Verification items for the finished model (mm, model axes). Face numbers are marked on the shaded views. A direction names the side the tool comes from. Coordinates: 2 decimals unless noted, no trailing zeros. Write each loop counter-clockwise with the first axis right and the second up, starting at its lowest first coordinate (ties: lowest second). Pieces come first, ordered by that corner, then holes. Notation, with made-up numbers: (-29, 44) -> (-2, 44) arc R15 cw to (-2, 73) -> close; hole circle Ø9 at (-36, -13). An arc over 180 degrees is marked (long way). Answer in a Markdown table with one row per item.
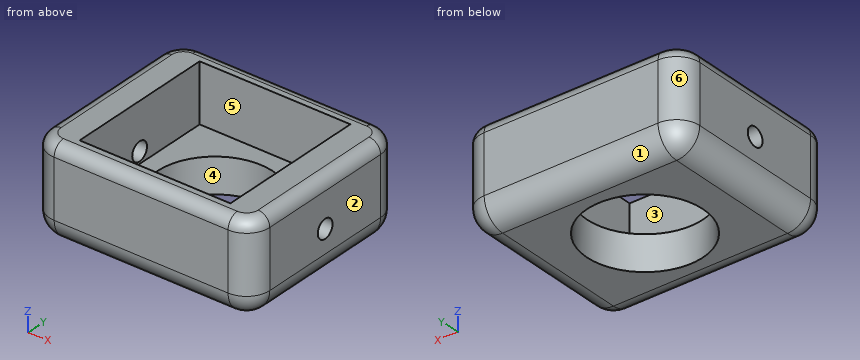
```python
from build123d import *

# Parameters (mm, degrees)
F0_W         = 19
F0_H         = 16
F0_W_2       = 13
F0_H_2       = 13
F0_R         = 5
F1_DEPTH     = 3
F2_W         = 19
F2_H         = 16
F2_W_2       = 13
F2_H_2       = 13
F3_DEPTH     = 5
F5_D         = 1.6
F6_R         = 2
F7_T1_DEPTH  = 11
F7_S5_W      = 2
F7_S5_H      = 2
F7_T6_DEPTH  = 2
F7_S11_W     = 2
F7_S11_H     = 2
F7_T12_DEPTH = 2
F7_S17_W     = 2
F7_S17_H     = 2
F7_T18_DEPTH = 2
F7_S23_W     = 2
F7_S23_H     = 2
F7_T24_DEPTH = 2
F8_R         = 1


# Not quite as in the source:
# - a fillet or chamfer that OpenCascade refuses, or shapes differently, is made with other operations: its cross-section is extruded or revolved along the edge and cut away or added


with BuildPart() as f1:
    # F0 (on Top) → F1 (new body)
    with BuildSketch(Plane.XY):
        Rectangle(F0_W, F0_H)
        Rectangle(F0_W_2, F0_H_2, mode=Mode.SUBTRACT)
        Rectangle(F0_W_2, F0_H_2)
        Circle(F0_R, mode=Mode.SUBTRACT)
    extrude(amount=F1_DEPTH)

    # F2 (on face) → F3 (join)
    with BuildSketch(Plane.XY.offset(3)):
        Rectangle(F2_W, F2_H)
        Rectangle(F2_W_2, F2_H_2, mode=Mode.SUBTRACT)
    extrude(amount=F3_DEPTH)

    # F5 (through all)
    with Locations(Plane.YZ.offset(9.5)):
        with Locations((0, 4)):
            Hole(F5_D / 2)

    # F6
    f6_edges = [f1.edges().sort_by_distance(p)[0] for p in [
        (0, -8, 0),
        (0, 8, 0),
        (-9.5, 0, 0),
        (9.5, 0, 0),
    ]]
    fillet(f6_edges, radius=F6_R)

    # F7: fillet of radius 2 on 4 edges, made by hand

    # F7_s2 → F7_t1 (cut)
    with BuildSketch(Plane.XY.offset(2)):
        with BuildLine():
            ThreePointArc((9.5, -6), (8.9142135624, -7.4142135624), (7.5, -8))
            Line((7.5, -8), (9.5, -8))
            Line((9.5, -8), (9.5, -6))
        make_face()
        with BuildLine():
            ThreePointArc((9.5, 6), (8.9142135624, 7.4142135624), (7.5, 8))
            Line((7.5, 8), (9.5, 8))
            Line((9.5, 8), (9.5, 6))
        make_face()
        with BuildLine():
            ThreePointArc((-7.5, -8), (-8.9142135624, -7.4142135624), (-9.5, -6))
            Line((-9.5, -6), (-9.5, -8))
            Line((-9.5, -8), (-7.5, -8))
        make_face()
        with BuildLine():
            ThreePointArc((-7.5, 8), (-8.9142135624, 7.4142135624), (-9.5, 6))
            Line((-9.5, 6), (-9.5, 8))
            Line((-9.5, 8), (-7.5, 8))
        make_face()
    extrude(amount=F7_T1_DEPTH, mode=Mode.SUBTRACT)


with BuildPart() as f7_tool4:
    # F7_s5 → F7_t6 (new body)
    with BuildSketch(Plane.XZ.offset(-6)):
        with Locations((-8.5, 1)):
            Rectangle(F7_S5_W, F7_S5_H)
    extrude(amount=-F7_T6_DEPTH)

    # F7_s7 → F7_t8 (revolve, cut)
    with BuildSketch(Plane(origin=(-7.5, 6, 2), x_dir=(0.7071067812, 0, 0.7071067812), z_dir=(-0.7071067812, 0, 0.7071067812))):
        with BuildLine():
            ThreePointArc((0, -2), (2, 0), (0, 2))
            Line((0, 2), (0, -2))
        make_face()
    revolve(axis=Axis((-7.5, 6, 2), (0, 1, 0)), mode=Mode.SUBTRACT)


with BuildPart() as f1_1:
    add(f1.part)

    # F7_t3: cut F7_tool4
    add(f7_tool4.part, mode=Mode.SUBTRACT)


with BuildPart() as f7_tool10:
    # F7_s11 → F7_t12 (new body)
    with BuildSketch(Plane.XZ.offset(6)):
        with Locations((-8.5, 1)):
            Rectangle(F7_S11_W, F7_S11_H)
    extrude(amount=F7_T12_DEPTH)

    # F7_s13 → F7_t14 (revolve, cut)
    with BuildSketch(Plane(origin=(-7.5, -6, 2), x_dir=(0.7071067812, 0, 0.7071067812), z_dir=(0.7071067812, 0, -0.7071067812))):
        with BuildLine():
            ThreePointArc((0, -2), (2, 0), (0, 2))
            Line((0, 2), (0, -2))
        make_face()
    revolve(axis=Axis((-7.5, -6, 2), (0, -1, 0)), mode=Mode.SUBTRACT)


with BuildPart() as f1_2:
    add(f1_1.part)

    # F7_t9: cut F7_tool10
    add(f7_tool10.part, mode=Mode.SUBTRACT)


with BuildPart() as f7_tool16:
    # F7_s17 → F7_t18 (new body)
    with BuildSketch(Plane.YZ.offset(7.5)):
        with Locations((7, 1)):
            Rectangle(F7_S17_W, F7_S17_H)
    extrude(amount=F7_T18_DEPTH)

    # F7_s19 → F7_t20 (revolve, cut)
    with BuildSketch(Plane(origin=(7.5, 6, 2), x_dir=(0, -0.7071067812, 0.7071067812), z_dir=(0, 0.7071067812, 0.7071067812))):
        with BuildLine():
            ThreePointArc((0, -2), (2, 0), (0, 2))
            Line((0, 2), (0, -2))
        make_face()
    revolve(axis=Axis((7.5, 6, 2), (1, 0, 0)), mode=Mode.SUBTRACT)


with BuildPart() as f1_3:
    add(f1_2.part)

    # F7_t15: cut F7_tool16
    add(f7_tool16.part, mode=Mode.SUBTRACT)


with BuildPart() as f7_tool22:
    # F7_s23 → F7_t24 (new body)
    with BuildSketch(Plane.YZ.offset(7.5)):
        with Locations((-7, 1)):
            Rectangle(F7_S23_W, F7_S23_H)
    extrude(amount=F7_T24_DEPTH)

    # F7_s25 → F7_t26 (revolve, cut)
    with BuildSketch(Plane(origin=(7.5, -6, 2), x_dir=(0, 0.7071067812, 0.7071067812), z_dir=(0, 0.7071067812, -0.7071067812))):
        with BuildLine():
            ThreePointArc((0, -2), (2, 0), (0, 2))
            Line((0, 2), (0, -2))
        make_face()
    revolve(axis=Axis((7.5, -6, 2), (1, 0, 0)), mode=Mode.SUBTRACT)


with BuildPart() as f1_4:
    add(f1_3.part)

    # F7_t21: cut F7_tool22
    add(f7_tool22.part, mode=Mode.SUBTRACT)

    # F8
    f8_edges = [f1_4.edges().sort_by_distance(p)[0] for p in [
        (0, 8, 8),
    ]]
    fillet(f8_edges, radius=F8_R)


solid = f1_4.part
```
1. Section check C-C, the plane x = 0. Record the boundary of the cut face in (y, z), plus the area to 3 significant figures.
Geometry says:
| item | result |
|---|---|
| outline | (-8, 2) arc R2 ccw to (-6, 0) -> (-5, 0) -> (-5, 3) -> (-6.5, 3) -> (-6.5, 8) -> (-7, 8) arc R1 ccw to (-8, 7) -> close; (5, 0) -> (6, 0) arc R2 ccw to (8, 2) -> (8, 7) arc R1 ccw to (7, 8) -> (6.5, 8) -> (6.5, 3) -> (5, 3) -> close |
| area | 30.9 mm^2 |
2. Tool access check on the marked faces 5 and 6. Record the directions out of +Z, -Z, +X, -X, +Y, -Y that give a thin tool (end or side, any length) a straight path to the whole face; none if there is none.
Geometry says:
| item | result |
|---|---|
| face 5 | +Z |
| face 6 | +Z, -Z, -X, +Y |
3. Thickness scan on line 1 (Y direction, x = -1.5, z = 5); line 2 (X direction, y = 1.75, z = 3.25); line 3 (Z direction, x = -1.25, y = 5). Record the ranges inside material, lowest first. Write a range as from..to.
Geometry says:
| item | result |
|---|---|
| line 1 | -8..-6.5, 6.5..8 |
| line 2 | -9.5..-6.5, 6.5..9.5 |
| line 3 | 0..3 |
4. Section check D-D, the plane y = -4. Record the boundary of the cut face in (x, z).
Geometry says:
| item | result |
|---|---|
| outline | (-9.5, 2) arc R2 ccw to (-7.5, 0) -> (-3, 0) -> (-3, 3) -> (-6.5, 3) -> (-6.5, 8) -> (-8.5, 8) arc R1 ccw to (-9.5, 7) -> close; (3, 0) -> (7.5, 0) arc R2 ccw to (9.5, 2) -> (9.5, 7) arc R1 ccw to (8.5, 8) -> (6.5, 8) -> (6.5, 3) -> (3, 3) -> close |
5. Depth check by flat-ended pin: P1, Ø9, axis at x = 0, y = 0, coming from the +Z side; P2, Ø6.5, axis at x = 2, y = -2.5, coming from the +Z side. Enter the tip coordinate at first touch or a pass-through.
Geometry says:
| item | result |
|---|---|
| P1 | through |
| P2 | z = 3 |
6. Section check A-A, the plane y = 0. Record the boundary of the cut face in (x, z).
Geometry says:
| item | result |
|---|---|
| outline | (-9.5, 2) arc R2 ccw to (-7.5, 0) -> (-5, 0) -> (-5, 3) -> (-6.5, 3) -> (-6.5, 3.2) -> (-9.5, 3.2) -> close; (-9.5, 4.8) -> (-6.5, 4.8) -> (-6.5, 8) -> (-8.5, 8) arc R1 ccw to (-9.5, 7) -> close; (5, 0) -> (7.5, 0) arc R2 ccw to (9.5, 2) -> (9.5, 3.2) -> (6.5, 3.2) -> (6.5, 3) -> (5, 3) -> close; (6.5, 4.8) -> (9.5, 4.8) -> (9.5, 7) arc R1 ccw to (8.5, 8) -> (6.5, 8) -> close |
7. Mould release check, pull along Y, two halves, no side actions. Record for the marked faces 1, 2, 3 and 4: released by +Y, released by -Y, zero draft, split by the parting line, or undercut.
Geometry says:
| item | result |
|---|---|
| face 1 | released by +Y |
| face 2 | zero draft |
| face 3 | undercut |
| face 4 | undercut |
8. Section check B-B, the plane z = 2.5. Record the boundary of the cut face in (x, y), plus the area to 3 significant figures.
Geometry says:
| item | result |
|---|---|
| outline | (-9.5, -6) arc R2 ccw to (-7.5, -8) -> (7.5, -8) arc R2 ccw to (9.5, -6) -> (9.5, 6) arc R2 ccw to (7.5, 8) -> (-7.5, 8) arc R2 ccw to (-9.5, 6) -> close; hole circle Ø10 at (0, 0) |
| area | 222 mm^2 |
